Build history of the part. All positions in model axes, mm. Give positions to 0.01 mm unless a question says otherwise; leave off trailing zeros. Order: outer loops, then holes, each group sorted by start corner. A loop starts at its lowest first (then second) coordinate and runs counter-clockwise, first axis right, second up. Notation, with made-up numbers: (16, 17.25) -> (45, 17.25) arc R20 cw to (45, 49.25) -> close; hole circle Ø7 at (14.25, -9). An arc over 180 degrees is marked (long way). One line per item, written item: value. Start each with the question number.
(1) Saw through at B-B on y = 1. Give the cut face in (x, z), plus the area to 3 significant figures.
(2) Saw through at C-C on x = 25. Give the cut face in (y, z), plus the area to 3 significant figures.
(3) Saw through at A-A on z = -39.5. Give the cut face in (x, y), plus the area to 3 significant figures.
(4) Probe line 1 (Z direction, x = 21.5, y = 0.9); line 2 (X direction, y = 1.3, z = -23); line 3 (X direction, y = 0.8, z = -57.75). List the from-to ranges inside material, lowest first.
```python
from build123d import *

# Parameters (mm, degrees)
SKETCH_1_W      = 43
SKETCH_1_H      = 65
SKETCH_1_R      = 2
SKETCH_1_W_2    = 27.8
SKETCH_1_H_2    = 21.8
EXTRUDE_1_DEPTH = 1.5


with BuildPart() as part:
    # Эскиз1 → Бобышка-Вытянуть1 (new body)
    with BuildSketch(Plane(origin=(0, 0, 0), x_dir=(1, 0, 0), z_dir=(0, 1, 0))):
        with Locations((21.5, 32.5)):
            Rectangle(SKETCH_1_W, SKETCH_1_H)
        with Locations((21.5, 7.25)):
            Circle(SKETCH_1_R, mode=Mode.SUBTRACT)
        with Locations((21.5, 57.75)):
            Circle(SKETCH_1_R, mode=Mode.SUBTRACT)
        with Locations((21.5, 32.5)):
            Rectangle(SKETCH_1_W_2, SKETCH_1_H_2, mode=Mode.SUBTRACT)
    extrude(amount=EXTRUDE_1_DEPTH)


solid = part.part
```
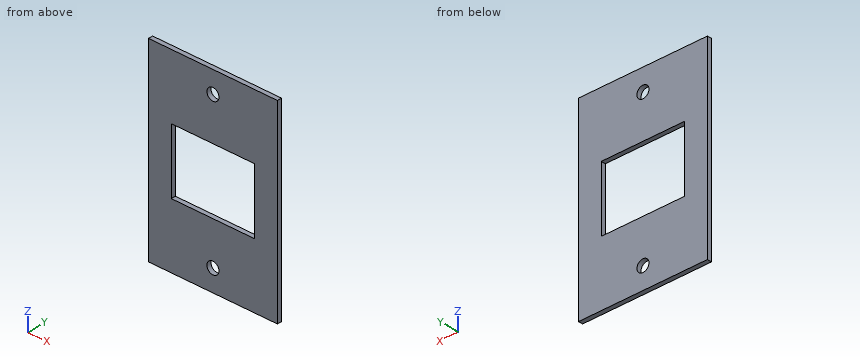
Results below:
1. outline: (0, -65) -> (43, -65) -> (43, 0) -> (0, 0) -> close; hole (7.6, -43.4) -> (35.4, -43.4) -> (35.4, -21.6) -> (7.6, -21.6) -> close; hole circle Ø4 at (21.5, -57.75); hole circle Ø4 at (21.5, -7.25)
1. area: 2,160 mm²
2. outline: (0, -65) -> (1.5, -65) -> (1.5, -43.4) -> (0, -43.4) -> close; (0, -21.6) -> (1.5, -21.6) -> (1.5, 0) -> (0, 0) -> close
2. area: 64.8 mm²
3. outline: (0, 0) -> (7.6, 0) -> (7.6, 1.5) -> (0, 1.5) -> close; (35.4, 0) -> (43, 0) -> (43, 1.5) -> (35.4, 1.5) -> close
3. area: 22.8 mm²
4. line 1: z = -65 to -59.75, -55.75 to -43.4, -21.6 to -9.25, -5.25 to 0
4. line 2: x = 0 to 7.6, 35.4 to 43
4. line 3: x = 0 to 19.5, 23.5 to 43
